Source: CAD feature listing. Evaluate the final solid. Frame: model axes, mm. Face numbers are marked on the shaded views. Give positions to 0.01 mm unless a question says otherwise; leave off trailing zeros. Order: outer loops, then holes, each group sorted by start corner. A loop starts at its lowest first (then second) coordinate and runs counter-clockwise, first axis right, second up. Notation, with made-up numbers: M -25.75,12.25 L -21.75,12.25 A26 ccw -21.75,33.25 Z; hole C 35,33 d3. An arc over 180 degrees is marked long. Use CSV: the item, a comma, the result in double quotes. Start each with the question number.
1. Mould query, pull axis X, two halves, no side actions, for the marked faces 1, 2 and 3. Classes: released by +X, released by -X, zero draft, split by the parting line, or undercut.
2. Section query B-B, the plane z = 9.75. Return the cut outline in (x, y), plus the area to 3 significant figures.
3. Section query A-A, the plane z = 3.5. Return the cut outline in (x, y), plus the area to 3 significant figures.
4. Section query C-C, the plane y = -8.5. State how many separate pieces and enclosed holes the cut face has, plus the area to 3 significant figures.
5. Line query: line 1 along Y through (x, z) = (16.75, 3.5); line 2 along Y through (x, z) = (15.75, 17.5); line 3 along Z through (x, y) = (12.25, 9.75). Output: solid intervals per line, ascending. Write a range as [from, to].
6. Pin query (flat end, axial travel): P1, Ø3, axis at x = 12.91, z = 9.75, coming from the -Y side; P2, Ø5.5, axis at y = 9, z = 3.5, coming from the +X side (3 decimals). Return the tip coordinate at first contact, or that it passes through.
from build123d import *

# Parameters (mm, degrees)
ESQUISSE1_W                                      = 14
ESQUISSE1_H                                      = 28
BOSS_EXTRU_1_DEPTH                               = 19.5
CHAMBRAGE_POUR_VIS_T_TE_RONDE_6_PANS_D           = 3.4
CHAMBRAGE_POUR_VIS_T_TE_RONDE_6_PANS_CBORE_D     = 6.5
CHAMBRAGE_POUR_VIS_T_TE_RONDE_6_PANS_CBORE_DEPTH = 1.65
TROU_TARAUD_M4X0_72_D                            = 3.3
TROU_TARAUD_M4X0_72_DEPTH                        = 11.5
TROU_TARAUD_M4X0_72_CSINK_D                      = 4.05
TROU_TARAUD_M4X0_72_CSINK_ANGLE                  = 90
TROU_TARAUD_M4X0_72_TIP                          = 0.991420021


with BuildPart() as part:
    # Esquisse1 → Boss.-Extru.1 (new body)
    with BuildSketch(Plane.XY):
        with Locations((14.905012229, -0.00220912)):
            Rectangle(ESQUISSE1_W, ESQUISSE1_H)
    extrude(amount=BOSS_EXTRU_1_DEPTH)

    # Chambrage pour Vis à tête ronde à 6 pans creux M31 (through all)
    with Locations(Plane(origin=(21.905012229, 0, 0), x_dir=(0, 0, -1), z_dir=(1, 0, 0))):
        with Locations((-3.5, 8.99779088), (-3.5, -9.00220912)):
            CounterBoreHole(CHAMBRAGE_POUR_VIS_T_TE_RONDE_6_PANS_D / 2, CHAMBRAGE_POUR_VIS_T_TE_RONDE_6_PANS_CBORE_D / 2, CHAMBRAGE_POUR_VIS_T_TE_RONDE_6_PANS_CBORE_DEPTH)

    # Trou taraudé M4x0.72
    with Locations(Plane.XY.offset(19.5)):
        with Locations((16.905012229, 7.99779088), (16.905012229, -8.00220912)):
            CounterSinkHole(TROU_TARAUD_M4X0_72_D / 2, TROU_TARAUD_M4X0_72_CSINK_D / 2, depth=TROU_TARAUD_M4X0_72_DEPTH, counter_sink_angle=TROU_TARAUD_M4X0_72_CSINK_ANGLE)
            with Locations((0, 0, -(TROU_TARAUD_M4X0_72_DEPTH + TROU_TARAUD_M4X0_72_TIP / 2))):  # 118° drill point
                Cone(0, TROU_TARAUD_M4X0_72_D / 2, TROU_TARAUD_M4X0_72_TIP, mode=Mode.SUBTRACT)

    # Esquisse15 → Trou taraudé M4x0.73 (revolve, cut)
    with BuildSketch(Plane(origin=(12.905012229, 13.99779088, 9.75), x_dir=(0, 0, 1), z_dir=(1, 0, 0))):
        Polygon((0, 0), (0, 28), (2.025, 28), (1.65, 27.625), (1.65, 0.375), (2.025, 0), align=None)
    revolve(axis=Axis((12.905012229, 20.34779088, 9.75), (0, -1, 0)), mode=Mode.SUBTRACT)


solid = part.part
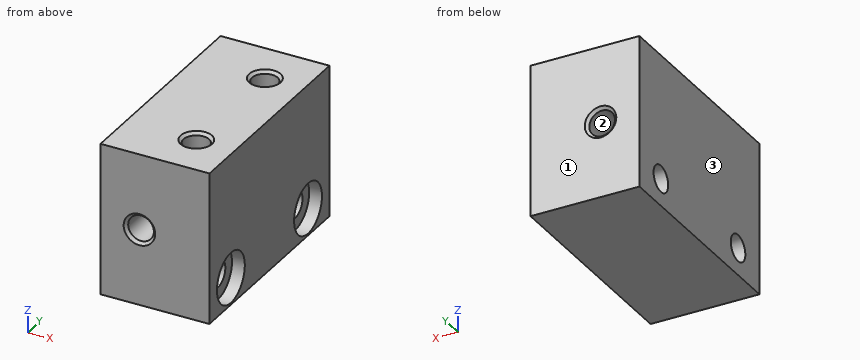
Result set:
1,face 1,"zero draft"
1,face 2,"undercut"
1,face 3,"released by -X"
2,outline,"M 7.91,-14 L 10.88,-14 L 11.26,-13.63 L 11.26,13.62 L 10.88,14 L 7.91,14 Z; M 14.56,-13.63 L 14.93,-14 L 21.91,-14 L 21.91,14 L 14.93,14 L 14.56,13.62 Z; hole C 16.91,-8 d3.3; hole C 16.91,8 d3.3"
2,area,"282 mm2"
3,outline,"M 7.91,-14 L 21.91,-14 L 21.91,-12.25 L 20.26,-12.25 L 20.26,-10.7 L 7.91,-10.7 Z; M 7.91,-7.3 L 20.26,-7.3 L 20.26,-5.75 L 21.91,-5.75 L 21.91,5.75 L 20.26,5.75 L 20.26,7.3 L 7.91,7.3 Z; M 7.91,10.7 L 20.26,10.7 L 20.26,12.25 L 21.91,12.25 L 21.91,14 L 7.91,14 Z"
3,area,"287 mm2"
4,separate pieces,"2"
4,enclosed holes,"1"
4,area,"176 mm2"
5,line 1,"[-14, -10.7], [-7.3, 7.3], [10.7, 14]"
5,line 2,"[-14, -9.18], [-6.82, 6.82], [9.18, 14]"
5,line 3,"[0, 1.98], [5.02, 8.24], [11.26, 19.5]"
6,P1,"through"
6,P2,"x = 20.255"
